Part model, mm, in its own coordinate system. A direction names the side the tool comes from. Give positions to 0.01 mm unless a question says otherwise; leave off trailing zeros. Loops run counter-clockwise (first coordinate to the right, second up) from the corner with the lowest first, then second, coordinate; pieces in that order, holes last. Notation, with made-up numbers: M -21,42.25 L -12,42.25 A19 ccw -12,53.25 Z; hole C 84,25 d1. An arc over 180 degrees is marked long. Put each result on its own line as item: value. Start each with the question number.
```python
from build123d import *

# Parameters (mm, degrees)
BOX_W             = 70
BOX_H             = 10
BOX_DEPTH         = 11
ARRAY_COUNT       = 8
CYLINDER001_R     = 20
CYLINDER001_DEPTH = 30
CYLINDER_R        = 30
CYLINDER_DEPTH    = 100


with BuildPart() as fusion:
    # Box → Box (new body)
    with BuildSketch(Plane(origin=(-35, -5, 90), x_dir=(1, 0, 0), z_dir=(0, 0, 1))):
        with Locations((35, 5)):
            Rectangle(BOX_W, BOX_H)
    extrude(amount=BOX_DEPTH)

    # Array: Fusion ×8 about axis
    array_axis = Axis((0, 0, 0), (0, 0, 1))


with BuildPart() as fusion_1:
    add(fusion.part)
    for i in range(1, ARRAY_COUNT):
        add(fusion.part.rotate(array_axis, i * 360 / ARRAY_COUNT))


with BuildPart() as obj1:
    # Cylinder001 → Cylinder001 (new body)
    with BuildSketch(Plane.XY.offset(80)):
        Circle(CYLINDER001_R)
    extrude(amount=CYLINDER001_DEPTH)


with BuildPart() as cut001:
    # Cylinder → Cylinder (new body)
    with BuildSketch(Plane.XY):
        Circle(CYLINDER_R)
    extrude(amount=CYLINDER_DEPTH)

    # Cut: cut obj1
    add(obj1.part, mode=Mode.SUBTRACT)

    # Cut001: cut Fusion
    add(fusion_1.part, mode=Mode.SUBTRACT)


solid = cut001.part
```
1) Wall check: L1, parallel to Y at x = 0, z = 88; L2, parallel to Z at x = 18, y = -14.5; L3, parallel to Z at x = -6, y = 15. Give the ranges that are in metal, low to high.
2) Band-saw the part on A-A on y = 0. Give the cut face in (x, z), then the cut area to 3 significant figures.
3) Band-saw the part on C-C on z = 75.5. Give the cut face in (x, y), then the cut area to 3 significant figures.
4) Pin check, flat tips, straight feed: pin 1 Ø4.5 at (x, y) = (-16, -16.5) entering from +Z; pin 2 Ø11.5 at (x, y) = (-14.5, 13.5) entering from +Z; pin 3 Ø4 at (y, z) = (-5, 69.5) entering from +X; pin 4 Ø11 at (x, z) = (-22, 93.5) entering from -Y. Stop position of each tip, or through.
5) Mould opens along X. For faces 1 (the cylindrical face through (27.712, -11.49, 49.3)), 2 (the flat face through (-20.89, -13.82, 94.93)), 3 (the flat face through (20.79, 13.72, 94.93)), 4 (the flat face through (10, 23, 100)) say: +X half, -X half, draft (parallel to the pull), parting line (faces both ways), or undercut.
6) Which spindle directions (+Z, -Z, +X, -X, +Y, -Y) get a long thin tool onto all of the face, cutting with end or side? Do faces 5 (the flat face through (-25, -5, 95)), 6 (the flat face through (17, -18, 90)), 7 (the flat face through (0, -25, 90)). Say none if no direction does.
7) Band-saw the part on D-D on x = -15. Give the cut face in (y, z).
8) Band-saw the part on B-B on x = -2.5. Give the cut face in (y, z), then the cut area to 3 significant figures.
Evaluation:
1. L1: -30 to -20, 20 to 30
1. L2: 0 to 90
1. L3: 0 to 80
2. outline: M -30,0 L 30,0 L 30,90 L 20,90 L 20,80 L -20,80 L -20,90 L -30,90 Z
2. area: 5,000 mm2
3. outline: C 0,0 d60
3. area: 2,830 mm2
4. pin 1: z = 90
4. pin 2: z = 100
4. pin 3: x = 29.85
4. pin 4: y = -25.05
5. face 1: parting line
5. face 2: undercut
5. face 3: undercut
5. face 4: draft
6. face 5: +Z, +X, -X
6. face 6: +Z
6. face 7: +Z, +Y, -Y
7. outline: M -25.98,0 L 25.98,0 L 25.98,100 L 22.07,100 L 22.07,90 L 13.23,90 L 13.23,80 L -13.23,80 L -13.23,90 L -22.07,90 L -22.07,100 L -25.98,100 Z
8. outline: M -29.9,0 L 29.9,0 L 29.9,90 L 19.84,90 L 19.84,80 L -19.84,80 L -19.84,90 L -29.9,90 Z
8. area: 4,980 mm2
